```python
from build123d import *

# Parameters (mm, degrees)
F0_W          = 50
F0_H          = 50
F1_DEPTH      = 10
F2_R          = 5
F3_R          = 5
F4_R          = 15
F4_R_2        = 7.5
F5_DEPTH      = 12.5
F5_DEPTH_BACK = 12.5
F6_DEPTH      = 5
F6_DEPTH_BACK = 5.25


with BuildPart() as f1:
    # F0 (on Top) → F1 (new body)
    with BuildSketch(Plane.XY):
        Rectangle(F0_W, F0_H)
    extrude(amount=F1_DEPTH)

    # F2
    f2_edges = [f1.edges().sort_by_distance(p)[0] for p in [
        (-25, -25, 5),
    ]]
    fillet(f2_edges, radius=F2_R)

    # F3
    f3_edges = [f1.edges().sort_by_distance(p)[0] for p in [
        (25, -25, 5),
        (-25, 25, 5),
        (25, 25, 5),
        (0, 25, 10),
        (25, 0, 10),
        (2.5, -25, 10),
        (-25, 2.5, 10),
    ]]
    fillet(f3_edges, radius=F3_R)

    # F4 (on Front) → F5 (join, two sides)
    with BuildSketch(Plane.XZ) as f5_sk:
        with Locations((0, 22.1625054122)):
            Circle(F4_R)
        with Locations((0, 22.1625054122)):
            Circle(F4_R_2, mode=Mode.SUBTRACT)
    extrude(amount=F5_DEPTH)
    extrude(f5_sk.sketch, amount=-F5_DEPTH_BACK)

    # F4 (on Front) → F6 (cut, two sides)
    with BuildSketch(Plane.XZ) as f6_sk:
        with Locations((0, 22.1625054122)):
            Circle(F4_R)
        with Locations((0, 22.1625054122)):
            Circle(F4_R_2, mode=Mode.SUBTRACT)
    extrude(amount=-F6_DEPTH, mode=Mode.SUBTRACT)
    extrude(f6_sk.sketch, amount=F6_DEPTH_BACK, mode=Mode.SUBTRACT)


solid = f1.part
```
For this review, take the finished solid that the model builds, in its own axes (mm). Coordinates: 2 decimals unless noted, no trailing zeros. Loops run counter-clockwise (first coordinate to the right, second up) from the corner with the lowest first, then second, coordinate; pieces in that order, holes last. Notation, with made-up numbers: (-23, 64) -> (-12, 64) arc R26 ccw to (-12, 103) -> close; hole circle Ø6 at (0.25, 72.25). An arc over 180 degrees is marked (long way). Return JSON: item names as keys, results as strings. Group by question number.
(1) Mouldability with a two-part tool opening along Y and no side actions: class faces 1 (the cylindrical face through (-24, 23, 3)), 2 (the flat face through (-7, -5.25, 19)), 3 (the flat face through (0, -12.5, 30)) as pulls with the +Y half, pulls with the -Y half, needs draft (parallel to the pull), parting line crosses it, or undercut.
(2) Consider section A-A, the plane x = 0. Give the boundary of the cut face in (y, z), plus the area to 3 significant figures.
(3) Consider section D-D, the plane z = 13. Give the boundary of the cut face in (x, y), plus the area to 3 significant figures.
(4) Consider section C-C, the plane y = 10. Give the boundary of the cut face in (x, z).
(5) To check wall thickness, follow L1, parallel to Y at x = 1, z = 13; L2, parallel to Z at x = 0, y = -10; L3, parallel to X at y = 8, z = 22. State the ranges of each line that lie inside material, in increasing order.
(6) For pin 1 Ø6 at (y, z) = (12, 27) entering from -X; pin 2 Ø15 at (x, z) = (-0.5, 20.5) entering from +Y; pin 3 Ø21.5 at (x, z) = (2, 30) entering from -Y; pin 4 Ø12 at (x, z) = (0, 22.16) entering from +Y, all flat-tipped, find the tip position at first contact; note any pin that passes through.
(7) Consider section B-B, the plane z = 21.5. Give the boundary of the cut face in (x, y), plus the area to 3 significant figures.
Results below:
{
 "1": {"face 1": "pulls with the +Y half", "face 2": "undercut", "face 3": "pulls with the -Y half"},
 "2": {"outline": "(-25, 0) -> (25, 0) -> (25, 5) arc R5 ccw to (20, 10) -> (12.5, 10) -> (12.5, 14.66) -> (5, 14.66) -> (5, 7.16) -> (-5.25, 7.16) -> (-5.25, 14.66) -> (-12.5, 14.66) -> (-12.5, 10) -> (-20, 10) arc R5 ccw to (-25, 5) -> close; (-12.5, 29.66) -> (-5.25, 29.66) -> (-5.25, 37.16) -> (-12.5, 37.16) -> close; (5, 29.66) -> (12.5, 29.66) -> (12.5, 37.16) -> (5, 37.16) -> close", "area": "640 mm2"},
 "3": {"outline": "(-11.88, -12.5) -> (11.88, -12.5) -> (11.88, -5.25) -> (-11.88, -5.25) -> close; (-11.88, 5) -> (11.88, 5) -> (11.88, 12.5) -> (-11.88, 12.5) -> close", "area": "350 mm2"},
 "4": {"outline": "(-25, 0) -> (25, 0) -> (25, 5) arc R5 ccw to (20, 10) -> (8.78, 10) arc R15 ccw (long way) to (-8.78, 10) -> (-20, 10) arc R5 ccw to (-25, 5) -> close; hole circle Ø15 at (0, 22.16)"},
 "5": {"L1": "y = -12.5 to -5.25, 5 to 12.5", "L2": "z = 0 to 14.66, 29.66 to 37.16", "L3": "x = -15 to -7.5, 7.5 to 15"},
 "6": {"pin 1": "stops at x = -14.89", "pin 2": "stops at y = 12.5", "pin 3": "stops at y = -12.5", "pin 4": "passes through"},
 "7": {"outline": "(-14.99, -12.5) -> (-7.47, -12.5) -> (-7.47, -5.25) -> (-14.99, -5.25) -> close; (-14.99, 5) -> (-7.47, 5) -> (-7.47, 12.5) -> (-14.99, 12.5) -> close; (7.47, -12.5) -> (14.99, -12.5) -> (14.99, -5.25) -> (7.47, -5.25) -> close; (7.47, 5) -> (14.99, 5) -> (14.99, 12.5) -> (7.47, 12.5) -> close", "area": "222 mm2"}
}
